Part model, mm, in its own coordinate system. A direction names the side the tool comes from. Coordinates: 2 decimals unless noted, no trailing zeros. Loops run counter-clockwise (first coordinate to the right, second up) from the corner with the lowest first, then second, coordinate; pieces in that order, holes last. Notation, with made-up numbers: M 18,36 L 40,36 A24 cw 40,65 Z; hole C -23.75,33 d6. An arc over 180 degrees is marked long. Use CSV: the item, a comma, the result in double quotes. Start each with the question number.
from build123d import *

# Parameters (mm, degrees)
SKETCH1_W           = 63.5
SKETCH1_H           = 25.4
SKETCH1_W_2         = 60.325
SKETCH1_H_2         = 22.225
BOSS_EXTRUDE1_DEPTH = 76.2
SKETCH2_W           = 12.7
SKETCH2_H           = 12.7
CUT_EXTRUDE1_DEPTH  = 515.310800975


with BuildPart() as part:
    # Sketch1 → Boss-Extrude1 (new body)
    with BuildSketch(Plane(origin=(0, 25.4, 0), x_dir=(1, 0, 0), z_dir=(0, 1, 0))):
        with Locations((298.45, -368.3)):
            Rectangle(SKETCH1_W, SKETCH1_H)
        with Locations((298.45, -368.3)):
            Rectangle(SKETCH1_W_2, SKETCH1_H_2, mode=Mode.SUBTRACT)
    extrude(amount=BOSS_EXTRUDE1_DEPTH)

    # Sketch2 → Cut-Extrude1 (cut, through all)
    with BuildSketch(Plane.XY):
        Polygon((266.7, 101.6), (317.5, 101.6), (266.7, 25.4), align=None)
        with Locations((323.85, 95.25)):
            Rectangle(SKETCH2_W, SKETCH2_H)
    extrude(amount=CUT_EXTRUDE1_DEPTH, mode=Mode.SUBTRACT)


solid = part.part
1. Slice it at C-C, the plane y = 94. List the corners of the cut face in (x, z), and give its area (3 significant figures).
2. Slice it at D-D, the plane y = 57.5. List the corners of the cut face in (x, z), and give its area (3 significant figures).
3. Pin check, flat tips, straight feed: pin 1 (0.5 mm diameter, centred on y = 94.5, z = 356.5, fed in from +X); pin 2 (5 mm diameter, centred on x = 289.5, z = 358.5, fed in from -Y); pin 3 (6 mm diameter, centred on y = 91.5, z = 363, fed in from -X); pin 4 (14 mm diameter, centred on x = 327, z = 366, fed in from +Y). Stop position of each tip, or through.
4. Two-plate mould, pull along Z, no slides. Class faces 4 (the face through (305, 54, 355.6)), 5 (the face through (305, 54, 357.188)), 6 (the face through (330.2, 57, 368)): pulls with the +Z half, pulls with the -Z half, needs draft (parallel to the pull), parting line crosses it, or undercut.
5. Wall check: probe 1 along Z at (x, y) = (314, 75); probe 2 along X at (y, z) = (43.5, 360.5); probe 3 along Y at (x, z) = (325, 357). Give the ranges that are in metal, low to high.
6. Slice it at B-B, the plane z = 367.75. List the corners of the cut face in (x, y), and give its area (3 significant figures).
7. Slice it at A-A, the plane x = 307.5. List the corners of the cut face in (y, z).
8. Tool access for faces 1 (the face through (317.5, 95, 380)), 2 (the face through (296, 25.4, 380)), 3 (the face through (268.287, 27, 368)): list every direction of +Z, -Z, +X, -X, +Y, -Y with a clear straight run to the whole face (end or side of a thin tool).
Found:
1,outline,"M 312.43,355.6 L 317.5,355.6 L 317.5,357.19 L 312.43,357.19 Z; M 312.43,379.41 L 317.5,379.41 L 317.5,381 L 312.43,381 Z"
1,area,"16.1 mm^2"
2,outline,"M 288.1,355.6 L 330.2,355.6 L 330.2,381 L 288.1,381 L 288.1,379.41 L 328.61,379.41 L 328.61,357.19 L 288.1,357.19 Z"
2,area,"169 mm^2"
3,pin 1,"x = 317.5"
3,pin 2,"y = 25.4"
3,pin 3,"x = 328.61"
3,pin 4,"y = 88.9"
4,face 4,"pulls with the -Z half"
4,face 5,"undercut"
4,face 6,"needs draft"
5,probe 1,"355.6 to 357.19, 379.41 to 381"
5,probe 2,"328.61 to 330.2"
5,probe 3,"25.4 to 88.9"
6,outline,"M 266.7,25.4 L 268.29,25.4 L 268.29,27.78 Z; M 328.61,25.4 L 330.2,25.4 L 330.2,88.9 L 328.61,88.9 Z"
6,area,"103 mm^2"
7,outline,"M 25.4,355.6 L 86.6,355.6 L 86.6,357.19 L 25.4,357.19 Z; M 25.4,379.41 L 86.6,379.41 L 86.6,381 L 25.4,381 Z"
8,face 1,"+Z, -Z, +X, +Y"
8,face 2,"+Z, -Z, +X, -X, -Y"
8,face 3,"+Y, -Y"
